```python
from build123d import *

# Parameters (mm, degrees)
BOSS_EXTRUDE1_DEPTH     = 5.25
CUT_EXTRUDE1_DEPTH      = 82.622208988
CUT_EXTRUDE1_DEPTH_BACK = 82.622208988
SKETCH2_R               = 4
SKETCH3_R               = 47
BOSS_EXTRUDE2_DEPTH     = 56.5
CUT_EXTRUDE4_DEPTH      = 103.213917839
CUT_EXTRUDE4_DEPTH_BACK = 103.213917839
SKETCH5_R               = 4
SKETCH5_R_2             = 15
CUT_EXTRUDE5_DEPTH      = 56.5
SKETCH6_R               = 42
BOSS_EXTRUDE3_DEPTH     = 36.5
CUT_EXTRUDE6_DEPTH      = 50.5
CUT_EXTRUDE6_DEPTH_BACK = 42.5
SKETCH7_R               = 39.5
SKETCH9_R               = 4.8
BOSS_EXTRUDE4_DEPTH     = 6
SKETCH10_R              = 2.2
CUT_EXTRUDE7_DEPTH      = 124.063743645
SKETCH11_R              = 4.8
CUT_EXTRUDE8_DEPTH      = 4
SKETCH12_R              = 4
CUT_EXTRUDE9_DEPTH      = 11
SKETCH13_R              = 3.5
CUT_EXTRUDE10_DEPTH     = 11.25


with BuildPart() as part:
    # Sketch1 → Boss-Extrude1 (new, symmetric)
    with BuildSketch(Plane(origin=(0, 0, 0), x_dir=(1, 0, 0), z_dir=(0, 1, 0))):
        with BuildLine():
            Line((-51, 37.85), (-51, -37.85))
            ThreePointArc((-51, -37.85), (0, -63.510806167), (51, -37.85))
            Line((51, -37.85), (51, 37.85))
            ThreePointArc((51, 37.85), (0, 63.510806167), (-51, 37.85))
        make_face()
    extrude(amount=BOSS_EXTRUDE1_DEPTH, both=True)

    # Sketch2 → Cut-Extrude1 (cut, two sides: drawn at the far end of the back side and taken through both)
    with BuildSketch(Plane(origin=(0, 0, 0), x_dir=(1, 0, 0), z_dir=(0, 1, 0)).offset(-CUT_EXTRUDE1_DEPTH_BACK)):
        with Locations(Location((35.603972242, 46.4, 0), (0, 0, 270))):
            Circle(SKETCH2_R)
        with Locations(Location((-35.603972242, -46.4, 0), (0, 0, 270))):
            Circle(SKETCH2_R)
        with BuildLine():
            Line((-3.832427429, 60.7), (3.832427429, 60.7))
            ThreePointArc((3.832427429, 60.7), (6.5, 55.45), (3.832427429, 50.2))
            Line((3.832427429, 50.2), (-3.832427429, 50.2))
            ThreePointArc((-3.832427429, 50.2), (-6.5, 55.45), (-3.832427429, 60.7))
        make_face()
        with BuildLine():
            Line((-35.991994178, 35.203747742), (-40.918867911, 29.33212827))
            ThreePointArc((-40.918867911, 29.33212827), (-46.655283834, 30.663284077), (-48.962334564, 36.081398172))
            Line((-48.962334564, 36.081398172), (-44.035460831, 41.953017644))
            ThreePointArc((-44.035460831, 41.953017644), (-38.299044908, 40.621861837), (-35.991994178, 35.203747742))
        make_face()
        with BuildLine():
            Line((48.962334564, 36.081398172), (44.035460831, 41.953017644))
            ThreePointArc((44.035460831, 41.953017644), (38.299044908, 40.621861837), (35.991994178, 35.203747742))
            Line((35.991994178, 35.203747742), (40.918867911, 29.33212827))
            ThreePointArc((40.918867911, 29.33212827), (46.655283834, 30.663284077), (48.962334564, 36.081398172))
        make_face()
        with BuildLine():
            Line((40.918867911, -29.33212827), (35.991994178, -35.203747742))
            ThreePointArc((35.991994178, -35.203747742), (38.299044908, -40.621861837), (44.035460831, -41.953017644))
            Line((44.035460831, -41.953017644), (48.962334564, -36.081398172))
            ThreePointArc((48.962334564, -36.081398172), (46.655283834, -30.663284077), (40.918867911, -29.33212827))
        make_face()
        with BuildLine():
            Line((-3.832427429, -50.2), (3.832427429, -50.2))
            ThreePointArc((3.832427429, -50.2), (6.5, -55.45), (3.832427429, -60.7))
            Line((3.832427429, -60.7), (-3.832427429, -60.7))
            ThreePointArc((-3.832427429, -60.7), (-6.5, -55.45), (-3.832427429, -50.2))
        make_face()
        with BuildLine():
            Line((-35.991994178, -35.203747742), (-40.918867911, -29.33212827))
            ThreePointArc((-40.918867911, -29.33212827), (-46.655283834, -30.663284077), (-48.962334564, -36.081398172))
            Line((-48.962334564, -36.081398172), (-44.035460831, -41.953017644))
            ThreePointArc((-44.035460831, -41.953017644), (-38.299044908, -40.621861837), (-35.991994178, -35.203747742))
        make_face()
        with BuildLine():
            Line((-29.217888815, -46.094553684), (-33.02145317, -54.251323767))
            ThreePointArc((-33.02145317, -54.251323767), (-26.840826504, -57.56033819), (-20.333144152, -60.167979432))
            Line((-20.333144152, -60.167979432), (-16.529579796, -52.011209348))
            Line((-16.529579796, -52.011209348), (-29.217888815, -46.094553684))
        make_face()
        with BuildLine():
            Line((20.333144152, -60.167979432), (16.529579796, -52.011209348))
            Line((16.529579796, -52.011209348), (29.217888815, -46.094553684))
            Line((29.217888815, -46.094553684), (33.02145317, -54.251323767))
            ThreePointArc((33.02145317, -54.251323767), (26.840826504, -57.56033819), (20.333144152, -60.167979432))
        make_face()
    extrude(amount=CUT_EXTRUDE1_DEPTH + CUT_EXTRUDE1_DEPTH_BACK, mode=Mode.SUBTRACT)

    # Sketch3 → Boss-Extrude2 (add)
    with BuildSketch(Plane(origin=(0, 5.25, 0), x_dir=(1, 0, 0), z_dir=(0, 1, 0))):
        with Locations(Location((0, 0, 0), (0, 0, 90))):
            Circle(SKETCH3_R)
    extrude(amount=BOSS_EXTRUDE2_DEPTH)

    # Sketch4 → Cut-Extrude4 (cut, two sides: drawn at the far end of the back side and taken through both)
    with BuildSketch(Plane(origin=(0, 0, 0), x_dir=(0, 0, -1), z_dir=(1, 0, 0)).offset(-CUT_EXTRUDE4_DEPTH_BACK)):
        with BuildLine():
            Line((-47, 53.746268605), (-47, 76.557383468))
            Line((-47, 76.557383468), (47, 76.557383468))
            Line((47, 76.557383468), (47, 53.746268605))
            ThreePointArc((47, 53.746268605), (0, 61.75), (-47, 53.746268605))
        make_face()
    extrude(amount=CUT_EXTRUDE4_DEPTH + CUT_EXTRUDE4_DEPTH_BACK, mode=Mode.SUBTRACT)

    # Sketch5 → Cut-Extrude5 (cut)
    with BuildSketch(Plane(origin=(0, 5.25, 0), x_dir=(1, 0, 0), z_dir=(0, 1, 0))):
        with Locations(Location((20, 18, 0), (0, 0, 90))):
            Circle(SKETCH5_R)
        with Locations(Location((-20, 18, 0), (0, 0, 90))):
            Circle(SKETCH5_R)
        with Locations(Location((0, 21.5, 0), (0, 0, 90))):
            Circle(SKETCH5_R_2)
    extrude(amount=CUT_EXTRUDE5_DEPTH, mode=Mode.SUBTRACT)

    # Sketch6 → Boss-Extrude3 (add)
    with BuildSketch(Plane(origin=(0, -5.25, 0), x_dir=(-1, 0, 0), z_dir=(0, -1, 0))):
        with Locations(Location((0, 0, 0), (0, 0, 90))):
            Circle(SKETCH6_R)
    extrude(amount=BOSS_EXTRUDE3_DEPTH)

    # Sketch7 → Cut-Extrude6 (cut, two sides: drawn at the far end of the back side and taken through both)
    with BuildSketch(Plane(origin=(0, 0, 0), x_dir=(1, 0, 0), z_dir=(0, 1, 0)).offset(-CUT_EXTRUDE6_DEPTH_BACK)):
        with Locations(Location((0, 0, 0), (0, 0, 90))):
            Circle(SKETCH7_R)
    extrude(amount=CUT_EXTRUDE6_DEPTH + CUT_EXTRUDE6_DEPTH_BACK, mode=Mode.SUBTRACT)

    # Sketch9 → Boss-Extrude4 (add)
    with BuildSketch(Plane(origin=(0, 50.5, 0), x_dir=(-1, 0, 0), z_dir=(0, -1, 0))):
        with Locations((-20, 18)):
            Circle(SKETCH9_R)
        with Locations((20, 18)):
            Circle(SKETCH9_R)
    extrude(amount=-BOSS_EXTRUDE4_DEPTH)

    # Sketch10 → Cut-Extrude7 (cut, through all)
    with BuildSketch(Plane(origin=(0, 50.5, 0), x_dir=(-1, 0, 0), z_dir=(0, -1, 0))):
        with Locations(Location((-20, 18, 0), (0, 0, 90))):
            Circle(SKETCH10_R)
        with Locations(Location((20, 18, 0), (0, 0, 270))):
            Circle(SKETCH10_R)
    extrude(amount=-CUT_EXTRUDE7_DEPTH, mode=Mode.SUBTRACT)

    # Sketch11 → Cut-Extrude8 (cut)
    with BuildSketch(Plane(origin=(0, 50.5, 0), x_dir=(-1, 0, 0), z_dir=(0, -1, 0))):
        with Locations(Location((-20, 18, 0), (0, 0, 90))):
            Circle(SKETCH11_R)
        with Locations(Location((20, 18, 0), (0, 0, 270))):
            Circle(SKETCH11_R)
    extrude(amount=-CUT_EXTRUDE8_DEPTH, mode=Mode.SUBTRACT)

    # Sketch12 → Cut-Extrude9 (cut)
    with BuildSketch(Plane(origin=(0, 61.75, 0), x_dir=(1, 0, 0), z_dir=(0, 1, 0))):
        with Locations(Location((-36.15, 0, 0), (0, 0, 270))):
            Circle(SKETCH12_R)
    extrude(amount=-CUT_EXTRUDE9_DEPTH, mode=Mode.SUBTRACT)

    # Sketch13 → Cut-Extrude10 (cut)
    with BuildSketch(Plane(origin=(0, 61.75, 0), x_dir=(1, 0, 0), z_dir=(0, 1, 0))):
        with Locations(Location((-36.15, 0, 0), (0, 0, 270))):
            Circle(SKETCH13_R)
    extrude(amount=-CUT_EXTRUDE10_DEPTH, mode=Mode.SUBTRACT)


solid = part.part
```
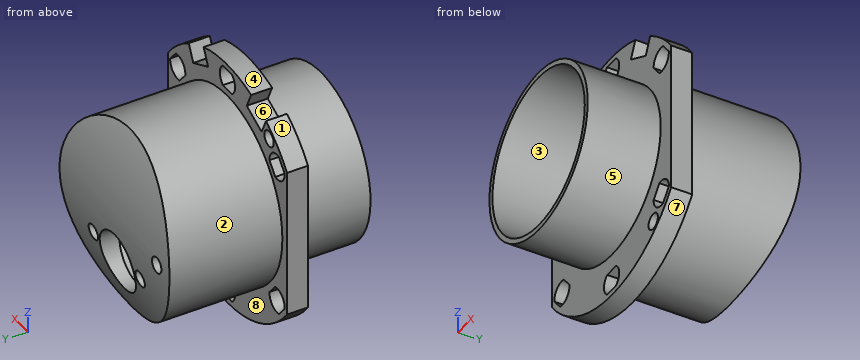
For this review, take the finished solid that the model builds, in its own axes (mm). Face numbers are marked on the shaded views. A direction names the side the tool comes from. Coordinates: 2 decimals unless noted, no trailing zeros. Order: outer loops, then holes, each group sorted by start corner. A loop starts at its lowest first (then second) coordinate and runs counter-clockwise, first axis right, second up. Notation, with made-up numbers: (-4, 12.5) -> (30, 12.5) arc R17 ccw to (30, 17.5) -> close; hole circle Ø2 at (-6, -26.75). An arc over 180 degrees is marked (long way). Use CSV: the item, a comma, the result in double quotes. Start each with the question number.
Item 1: Wall thickness on probe 1 along X at (y, z) = (58, 0); probe 2 along X at (y, z) = (55.8, -18); probe 3 along X at (y, z) = (57, -18): over which ranges is each line inside the solid? List them lowest first.
Item 2: We need section C-C, the plane x = -27.5. Give the boundary of the cut face in (y, z).
Item 3: We need section B-B, the plane y = -18.5. Give the boundary of the cut face in (x, z).
Item 4: We need section A-A, the plane z = 14. Give the boundary of the cut face in (x, y).
Item 5: Draft analysis for pull direction X (two halves, no side actions). For the marked faces 1, 2 and 3, state which applies: pulls with the +X half, pulls with the -X half, needs draft (parallel to the pull), parting line crosses it, or undercut.
Item 6: We need section D-D, the plane z = -18. Give the number of separate pieces and of enclosed holes in the cut face, then the cut area to 3 significant figures.
Item 7: Insertion check: pin 1 (3 mm diameter, centred on x = 13, y = 33.5, fed in from -Z); pin 2 (3 mm diameter, centred on x = -34.5, y = 4.5, fed in from +Z); pin 3 (8 mm diameter, centred on y = 36, z = -38, fed in from +X); pin 4 (8.5 mm diameter, centred on x = 0.5, y = 1.5, fed in from +Z). Each pin has a flat end and moves straight along its axis. Give the tip position at first contact, or say it passes through.
Item 8: For the marked faces 4, 5, 6, 7 and 8, list the 3-axis set-ups (+Z, -Z, +X, -X, +Y, -Y) from which the entire face can be reached by the end or side of a thin tool; tool diameter is ignored.
Derived:
1,probe 1,"x = -47 to -40.15, -32.15 to 47"
1,probe 2,"x = -43.42 to -22.2, -17.8 to -14.59, 14.59 to 17.8, 22.2 to 43.42"
1,probe 3,"x = -43.42 to -24, -16 to -14.59, 14.59 to 16, 24 to 43.42"
2,outline,"(-41.75, -31.75) -> (-5.25, -31.75) -> (-5.25, -57.25) -> (5.25, -57.25) -> (5.25, -38.11) -> (56.54, -38.11) arc R142 ccw to (56.54, 38.11) -> (5.25, 38.11) -> (5.25, 46.9) -> (-5.25, 46.9) -> (-5.25, 31.75) -> (-41.75, 31.75) -> (-41.75, 28.35) -> (50.5, 28.35) -> (50.5, -28.35) -> (-41.75, -28.35) -> close"
3,outline,"circle Ø84 at (0, 0); hole circle Ø79 at (0, 0)"
4,outline,"(-51, -5.25) -> (-39.6, -5.25) -> (-39.6, -41.75) -> (-36.94, -41.75) -> (-36.94, 50.5) -> (36.94, 50.5) -> (36.94, -41.75) -> (39.6, -41.75) -> (39.6, -5.25) -> (51, -5.25) -> (51, 5.25) -> (44.87, 5.25) -> (44.87, 61.06) -> (-44.87, 61.06) -> (-44.87, 5.25) -> (-51, 5.25) -> close"
5,face 1,"pulls with the -X half"
5,face 2,"parting line crosses it"
5,face 3,"undercut"
6,separate pieces,"4"
6,enclosed holes,"0"
6,area,"1,710 mm^2"
7,pin 1,"stops at z = -45.57"
7,pin 2,"stops at z = 54.25"
7,pin 3,"stops at x = 32.45"
7,pin 4,"stops at z = 63.51"
8,face 4,"+Z, +Y, -Y"
8,face 5,"-Y"
8,face 6,"+Y, -Y"
8,face 7,"-Z, +Y, -Y"
8,face 8,"+Y"
